For this review, take the finished solid that the model builds, in its own axes (mm). A direction names the side the tool comes from. Round coordinates to 2 decimals unless told otherwise and drop trailing zeros. Order: outer loops, then holes, each group sorted by start corner. A loop starts at its lowest first (then second) coordinate and runs counter-clockwise, first axis right, second up. Notation, with made-up numbers: (52.5, 68) -> (65.5, 68) arc R16 cw to (65.5, 94) -> close; hole circle Ø3 at (-27, -25.75). An arc over 180 degrees is marked (long way). Answer in a Markdown table with one row per item.
```python
from build123d import *

# Parameters (mm, degrees)
BOSS_EXTRUDE1_DEPTH              = 6.35
FILLET1_R                        = 25.4
SKETCH11_R                       = 14.2875
CUT_EXTRUDE1_DEPTH               = 88.298066989
F_1_4_CLEARANCE_HOLE1_D          = 6.7564
BOSS_EXTRUDE2_DEPTH              = 12.7
FILLET2_R                        = 25
SKETCH25_W                       = 25
SKETCH25_H                       = 12.7
BOSS_EXTRUDE3_DEPTH              = 12
TAP_DRILL_FOR_10_32_TAP1_D       = 4.0386
TAP_DRILL_FOR_10_32_TAP1_DEPTH   = 25.4
TAP_DRILL_FOR_10_32_TAP1_TIP     = 1.213317848
FILLET4_R                        = 19.05
BOSS_EXTRUDE4_DEPTH              = 12.7
FILLET3_R                        = 3.175
F_3_32_0_09375_DOWEL_HOLE2_D     = 2.38125
F_3_32_0_09375_DOWEL_HOLE2_DEPTH = 8.128
F_3_32_0_09375_DOWEL_HOLE2_TIP   = 0.715399675


with BuildPart() as part:
    # Sketch2 → Boss-Extrude1 (new, symmetric)
    with BuildSketch(Plane(origin=(0, 0, 0), x_dir=(1, 0, 0), z_dir=(0, 1, 0))):
        Polygon((25.4, -82.55), (25.4, 0), (25.4, 57.15), (-25.4, 57.15), (-25.4, 0), (-25.4, -82.55), align=None)
    extrude(amount=BOSS_EXTRUDE1_DEPTH, both=True)

    # Fillet1
    fillet1_edges = [part.edges().sort_by_distance(p)[0] for p in [
        (25.4, 0, 82.55),
        (-25.4, 0, 82.55),
    ]]
    fillet(fillet1_edges, radius=FILLET1_R - 0.0001)  # a hair under: the kernel refuses the full size

    # Sketch11 → Cut-Extrude1 (cut, through all)
    with BuildSketch(Plane(origin=(0, 6.35, 0), x_dir=(1, 0, 0), z_dir=(0, 1, 0))):
        with Locations(Location((0, -57.15, 0), (0, 0, 270))):
            Circle(SKETCH11_R)
    extrude(amount=-CUT_EXTRUDE1_DEPTH, mode=Mode.SUBTRACT)

    # 1/4 Clearance Hole1 (through all)
    with Locations(Plane(origin=(0, 6.35, 0), x_dir=(1, 0, 0), z_dir=(0, 1, 0))):
        with Locations((-19.05, 50.8), (19.05, 50.8), (0, 38.1)):
            Hole(F_1_4_CLEARANCE_HOLE1_D / 2)

    # Sketch15 → Boss-Extrude2 (add)
    with BuildSketch(Plane.XZ.offset(6.35)):
        with BuildLine():
            Line((-4.225282002, 82.196097341), (-49.275251792, 74.59615776))
            Line((-49.275251792, 74.59615776), (-40.724748208, 51.10384224))
            Line((-40.724748208, 51.10384224), (-25.4, 42.256094737))
            Line((-25.4, 42.256094737), (-25.4, 57.15))
            ThreePointArc((-25.4, 57.15), (-19.396934846, 73.54874747), (-4.225282002, 82.196097341))
        make_face()
    extrude(amount=-BOSS_EXTRUDE2_DEPTH)

    # Fillet2
    fillet2_edges = [part.edges().sort_by_distance(p)[0] for p in [
        (-25.4, 0, 42.256094737),
    ]]
    fillet(fillet2_edges, radius=FILLET2_R)

    # Sketch25 → Boss-Extrude3 (add)
    with BuildSketch(Plane(origin=(-19.536399336, 0, -7.110667843), x_dir=(-0.34202014332566627, 0, 0.9396926207859093), z_dir=(-0.9396926207859093, 0, -0.34202014332566627))):
        with Locations((74.450587666, 0)):
            Rectangle(SKETCH25_W, SKETCH25_H)
    extrude(amount=BOSS_EXTRUDE3_DEPTH)

    # Tap Drill for #10-32 Tap1
    with Locations(Plane(origin=(-30.812710785, 0, -11.214909563), x_dir=(-0.3420201433256665, 0, 0.9396926207859093), z_dir=(-0.9396926207859092, 0, -0.34202014332566644))):
        with Locations((74.450587666, 0)):
            Hole(TAP_DRILL_FOR_10_32_TAP1_D / 2, depth=TAP_DRILL_FOR_10_32_TAP1_DEPTH)
            with Locations((0, 0, -(TAP_DRILL_FOR_10_32_TAP1_DEPTH + TAP_DRILL_FOR_10_32_TAP1_TIP / 2))):  # 118° drill point
                Cone(0, TAP_DRILL_FOR_10_32_TAP1_D / 2, TAP_DRILL_FOR_10_32_TAP1_TIP, mode=Mode.SUBTRACT)

    # Fillet4
    fillet4_edges = [part.edges().sort_by_distance(p)[0] for p in [
        (-40.724748208, 0, 51.10384224),
    ]]
    fillet(fillet4_edges, radius=FILLET4_R)

    # Sketch26 → Boss-Extrude4 (add)
    with BuildSketch(Plane.XZ.offset(6.35)):
        Polygon((-27.422249839, 82.55), (0, 82.55), (-49.275251792, 74.59615776), align=None)
    extrude(amount=-BOSS_EXTRUDE4_DEPTH)

    # Fillet3
    fillet3_edges = [part.edges().sort_by_distance(p)[0] for p in [
        (-60.551563241, 0, 70.49191604),
        (-52.001059658, 0, 46.99960052),
        (-27.422249839, 0, 82.55),
    ]]
    fillet(fillet3_edges, radius=FILLET3_R)

    # 3/32 (0.09375) Dowel Hole2
    with Locations(Plane(origin=(0, 6.35, 0), x_dir=(1, 0, 0), z_dir=(0, 1, 0))):
        with Locations((19.05, 38.1), (0, 50.8), (-19.05, 38.1), (0, 38.1)):
            Hole(F_3_32_0_09375_DOWEL_HOLE2_D / 2, depth=F_3_32_0_09375_DOWEL_HOLE2_DEPTH)
            with Locations((0, 0, -(F_3_32_0_09375_DOWEL_HOLE2_DEPTH + F_3_32_0_09375_DOWEL_HOLE2_TIP / 2))):  # 118° drill point
                Cone(0, F_3_32_0_09375_DOWEL_HOLE2_D / 2, F_3_32_0_09375_DOWEL_HOLE2_TIP, mode=Mode.SUBTRACT)


solid = part.part
```
Q1. Tool access review of faces 5 (the face through (-25.4, 0, -15)), 6 (the face through (-18.61, -0.09, -54.15)): name each direction out of +Z, -Z, +X, -X, +Y, -Y from which nothing blocks a thin tool from reaching the whole face with its end or side.
Answer key:
| item | result |
|---|---|
| face 5 | -Z, -X, +Y, -Y |
| face 6 | +Y, -Y |
Q2. Take a section at A-A, the plane x = 8.5. Write out the cut boundary in (y, z).
Answer key:
| item | result |
|---|---|
| outline | (-6.35, -57.15) -> (6.35, -57.15) -> (6.35, 45.67) -> (-6.35, 45.67) -> close; (-6.35, 68.63) -> (6.35, 68.63) -> (6.35, 81.09) -> (-6.35, 81.09) -> close |
Q3. To check wall thickness, follow probe 1 along X at (y, z) = (1.5, -38.1); probe 2 along X at (y, z) = (-1.5, -50.8); probe 3 along Z at (x, y) = (-19.05, 3). State the ranges of each line that lie inside material, in increasing order.
Answer key:
| item | result |
|---|---|
| probe 1 | x = -25.4 to -20.24, -17.86 to -3.38, 3.38 to 17.86, 20.24 to 25.4 |
| probe 2 | x = -25.4 to -22.43, -15.67 to -1.19, 1.19 to 15.67, 22.43 to 25.4 |
| probe 3 | z = -57.15 to -54.18, -47.42 to -39.29, -36.91 to 82.55 |
Q4. Take a section at B-B, the plane x = -12.5. Write out the cut boundary in (y, z).
Answer key:
| item | result |
|---|---|
| outline | (-6.35, -57.15) -> (6.35, -57.15) -> (6.35, 50.23) -> (-6.35, 50.23) -> close; (-6.35, 64.07) -> (6.35, 64.07) -> (6.35, 82.55) -> (-6.35, 82.55) -> close |
Q5. The part is to be moulded in two halves that separate along Y. For faces 1 (the face through (-7, 6.35, 14)), 2 (the face through (-43.52, 0.61, 61.34)), 3 (the face through (0, 0, -57.15)), 4 (the face through (-31.37, -0.21, 67.51)), say which applies: +Y half, -Y half, draft (parallel to the pull), parting line (faces both ways), or undercut.
Answer key:
| item | result |
|---|---|
| face 1 | +Y half |
| face 2 | undercut |
| face 3 | draft |
| face 4 | undercut |
Q6. Clearance check with flat-ended pins moving along their axes: pin 1 Ø6.5 at (y, z) = (2, -15.5) entering from -X; pin 2 Ø1.4 at (x, z) = (-19.05, -38.1) entering from +Y. State where each tip first meets the part, or that it passes through.
Answer key:
| item | result |
|---|---|
| pin 1 | stops at x = -25.4 |
| pin 2 | stops at y = -2.07 |
